Source: CAD feature listing. Evaluate the final solid. Frame: model axes, mm. A direction names the side the tool comes from. Give positions to 0.01 mm unless a question says otherwise; leave off trailing zeros. Write each loop counter-clockwise with the first axis right and the second up, starting at its lowest first coordinate (ties: lowest second). Pieces come first, ordered by that corner, then holes.
```python
from build123d import *

# Parameters (mm, degrees)
MODEL_W             = 69
MODEL_H             = 150
MODEL_W_2           = 45
MODEL_H_2           = 17.549304405
MODEL_H_3           = 17.549304404
BOSS_EXTRUDE1_DEPTH = 5.6
FILLET1_R           = 10
FILLET2_R           = 5


with BuildPart() as part:
    # Model → Boss-Extrude1 (new body)
    with BuildSketch(Plane.XY):
        with Locations((80.965167, 148.011716788)):
            Rectangle(MODEL_W, MODEL_H)
        with Locations((80.965167, 159.786368991)):
            Rectangle(MODEL_W_2, MODEL_H_2, mode=Mode.SUBTRACT)
        with Locations((80.965167, 183.335673395)):
            Rectangle(MODEL_W_2, MODEL_H_3, mode=Mode.SUBTRACT)
        with Locations((80.965167, 136.237064586)):
            Rectangle(MODEL_W_2, MODEL_H_3, mode=Mode.SUBTRACT)
        with Locations((80.965167, 112.687760182)):
            Rectangle(MODEL_W_2, MODEL_H_3, mode=Mode.SUBTRACT)
        Polygon((105.926079426, 198.110325597), (106.146551371, 198.108293598), (106.462865959, 198.106261598), (107.414180388, 198.293544218), (108.520604111, 198.844893414), (109.398766558, 199.71425053), (109.885769103, 200.555498319), (109.984998412, 200.855218244), (112.087101886, 207.226891318), (112.190056527, 207.542867239), (112.252032512, 209.101410849), (111.70865689, 210.547690825), (111.515176602, 210.816482466), (111.320006162, 211.085959339), (110.098534463, 212.052809224), (108.599544612, 212.48043722), (108.269000143, 212.479948671), (105.948092754, 212.479948671), (105.560658184, 212.469111341), (104.397338475, 212.149410087), (103.133434791, 211.291228969), (102.278640338, 210.021906619), (101.96638975, 208.85858691), (101.96638975, 208.469120341), (101.96638975, 202.110316597), (101.96638975, 201.723898027), (102.276947005, 200.56633565), (103.123952127, 199.298706633), (104.382775812, 198.437138849), (105.53830619, 198.113373596), align=None, mode=Mode.SUBTRACT)
        Polygon((56.006286573, 198.110325597), (55.786153295, 198.108293598), (55.468145374, 198.106261598), (54.515814946, 198.293544218), (53.410068555, 198.844893414), (52.531906108, 199.71425053), (52.046596896, 200.555498319), (51.947367588, 200.855218244), (49.84560278, 207.226891318), (49.740954806, 207.542867239), (49.678301488, 209.101410849), (50.213056021, 210.56377315), (50.409482639, 210.831658417), (50.604215924, 211.100221016), (51.829850284, 212.061356776), (53.331159242, 212.481980671), (53.663729825, 212.479948671), (55.983959888, 212.479948671), (56.37003558, 212.481751973), (57.534497197, 212.167486259), (58.804766127, 211.315229016), (59.662770703, 210.049900432), (59.982483497, 208.888061364), (59.965637583, 208.469120341), (59.965637583, 202.110316597), (59.965637583, 201.723898027), (59.653386995, 200.56633565), (58.806381873, 199.298706633), (57.547896854, 198.437138849), (56.392366477, 198.113373596), align=None, mode=Mode.SUBTRACT)
        Polygon((105.926079426, 97.910059981), (106.146551371, 97.911753313), (106.462865959, 97.915478646), (107.414180388, 97.727857359), (108.520604111, 97.177185497), (109.398766558, 96.307828381), (109.885769103, 95.466580591), (109.984998412, 95.164828667), (112.087101886, 88.792816927), (112.190056527, 88.478534338), (112.252032512, 86.922700061), (111.709769882, 85.473734765), (111.516141042, 85.203024117), (111.320811964, 84.933999869), (110.098774764, 83.968201755), (108.599536956, 83.541110091), (108.268994213, 83.541452906), (105.948092754, 83.541452906), (105.560658184, 83.55296757), (104.397338475, 83.872330157), (103.133434791, 84.732543275), (102.278640338, 86.002204291), (101.96638975, 87.164846667), (101.96638975, 87.55092657), (101.96638975, 93.910068981), (101.96638975, 94.29750355), (102.276947005, 95.457097927), (103.123952127, 96.723372277), (104.382775812, 97.584940062), (105.53830619, 97.906334648), align=None, mode=Mode.SUBTRACT)
        Polygon((56.006286573, 97.910059981), (55.786153295, 97.911753313), (55.468145374, 97.915478646), (54.515814946, 97.727857359), (53.410068555, 97.177185497), (52.531906108, 96.307828381), (52.046596896, 95.466580591), (51.947367588, 95.164828667), (49.84560278, 88.792816927), (49.740954806, 88.478534338), (49.678301488, 86.922700061), (50.213056021, 85.459660426), (50.409482639, 85.189743161), (50.604215924, 84.921519228), (51.829850284, 83.960722135), (53.331159242, 83.539759573), (53.663729825, 83.541452906), (55.983953956, 83.541452906), (56.37003894, 83.541906995), (57.534315492, 83.856513857), (58.804094924, 84.711544578), (59.661361982, 85.977712552), (59.980393619, 87.139060758), (59.981971512, 87.525137437), (59.981971512, 93.884279847), (59.981971512, 94.271714417), (59.653386995, 95.457097927), (58.806381873, 96.723372277), (57.547896854, 97.584940062), (56.392366477, 97.906334648), align=None, mode=Mode.SUBTRACT)
    extrude(amount=BOSS_EXTRUDE1_DEPTH)

    # Fillet1
    fillet1_edges = [part.edges().sort_by_distance(p)[0] for p in [
        (115.465167, 73.011716788, 2.8),
        (46.465167, 73.011716788, 2.8),
        (46.465167, 223.011716788, 2.8),
        (115.465167, 223.011716788, 2.8),
    ]]
    fillet(fillet1_edges, radius=FILLET1_R)

    # Fillet2
    fillet2_edges = [part.edges().sort_by_distance(p)[0] for p in [
        (58.465167, 192.110325597, 2.8),
        (58.465167, 174.561021193, 2.8),
        (103.465167, 174.561021193, 2.8),
        (103.465167, 192.110325597, 2.8),
        (58.465167, 168.561021193, 2.8),
        (58.465167, 151.011716788, 2.8),
        (103.465167, 151.011716788, 2.8),
        (103.465167, 168.561021193, 2.8),
        (58.465167, 127.462412384, 2.8),
        (103.465167, 127.462412384, 2.8),
        (103.465167, 145.011716788, 2.8),
        (58.465167, 145.011716788, 2.8),
        (58.465167, 103.91310798, 2.8),
        (103.465167, 103.91310798, 2.8),
        (103.465167, 121.462412384, 2.8),
        (58.465167, 121.462412384, 2.8),
    ]]
    fillet(fillet2_edges, radius=FILLET2_R)


solid = part.part
```
1. Cut plane D-D, the plane z = 4.45. State how many separate pieces and enclosed holes the cut face has, then the cut area to 3 significant figures.
2. Line query: L1, parallel to Y at x = 87.5, z = 4.35; L2, parallel to Y at x = 53.5, z = 4.7; L3, parallel to X at y = 89, z = 3.1. Output: solid intervals per line, ascending.
3. Access query for faces 4 (the cylindrical face through (49.317, 220.005, 2.839)), 5 (the flat face through (81, 174.561, 3)). Directions: +Z, -Z, +X, -X, +Y, -Y. A direction counts if a zero-diameter tool reaches every point of the face in a straight line with its end or side. Return the directions, or none.
4. Cut plane A-A, the plane y = 138.5. Return the cut outline in (x, z), then the cut area to 3 significant figures.
5. Mould query, pull axis X, two halves, no side actions, for faces 1 (the flat face through (46.465, 147, 3)), 2 (the flat face through (81, 223.012, 3)), 3 (the flat face through (58.465, 160, 3)). Classes: +X half, -X half, draft (parallel to the pull), parting line (faces both ways), or undercut.
6. Cut plane C-C, the plane y = 91. Return the cut outline in (x, z).
7. Cut plane B-B, the plane x = 66. Return the cut outline in (y, z).
8. Contact query for flat-ended pins moving along their axis: P1, Ø0.7, axis at x = 55.5, z = 2.5, coming from the -Y side; P2, Ø1.2, axis at x = 107, z = 3.5, coming from the -Y side. Output: stop coordinate, or through.
Response values:
1. separate pieces: 1
1. enclosed holes: 8
1. area: 6,710 mm2
2. L1: y = 73.01 to 103.91, 121.46 to 127.46, 145.01 to 151.01, 168.56 to 174.56, 192.11 to 223.01
2. L2: y = 73.46 to 83.54, 97.22 to 198.8, 212.48 to 222.56
2. L3: x = 46.47 to 49.91, 59.98 to 101.97, 112.02 to 115.47
3. face 4: +Z, -Z, -X, +Y
3. face 5: +Z, -Z
4. outline: (46.47, 0) - (58.47, 0) - (58.47, 5.6) - (46.47, 5.6) - close; (103.47, 0) - (115.47, 0) - (115.47, 5.6) - (103.47, 5.6) - close
4. area: 134 mm2
5. face 1: -X half
5. face 2: draft
5. face 3: undercut
6. outline: (46.47, 0) - (50.57, 0) - (50.57, 5.6) - (46.47, 5.6) - close; (59.98, 0) - (101.97, 0) - (101.97, 5.6) - (59.98, 5.6) - close; (111.36, 0) - (115.47, 0) - (115.47, 5.6) - (111.36, 5.6) - close
7. outline: (73.01, 0) - (103.91, 0) - (103.91, 5.6) - (73.01, 5.6) - close; (121.46, 0) - (127.46, 0) - (127.46, 5.6) - (121.46, 5.6) - close; (145.01, 0) - (151.01, 0) - (151.01, 5.6) - (145.01, 5.6) - close; (168.56, 0) - (174.56, 0) - (174.56, 5.6) - (168.56, 5.6) - close; (192.11, 0) - (223.01, 0) - (223.01, 5.6) - (192.11, 5.6) - close
8. P1: stops at y = 73.03
8. P2: stops at y = 73.06
